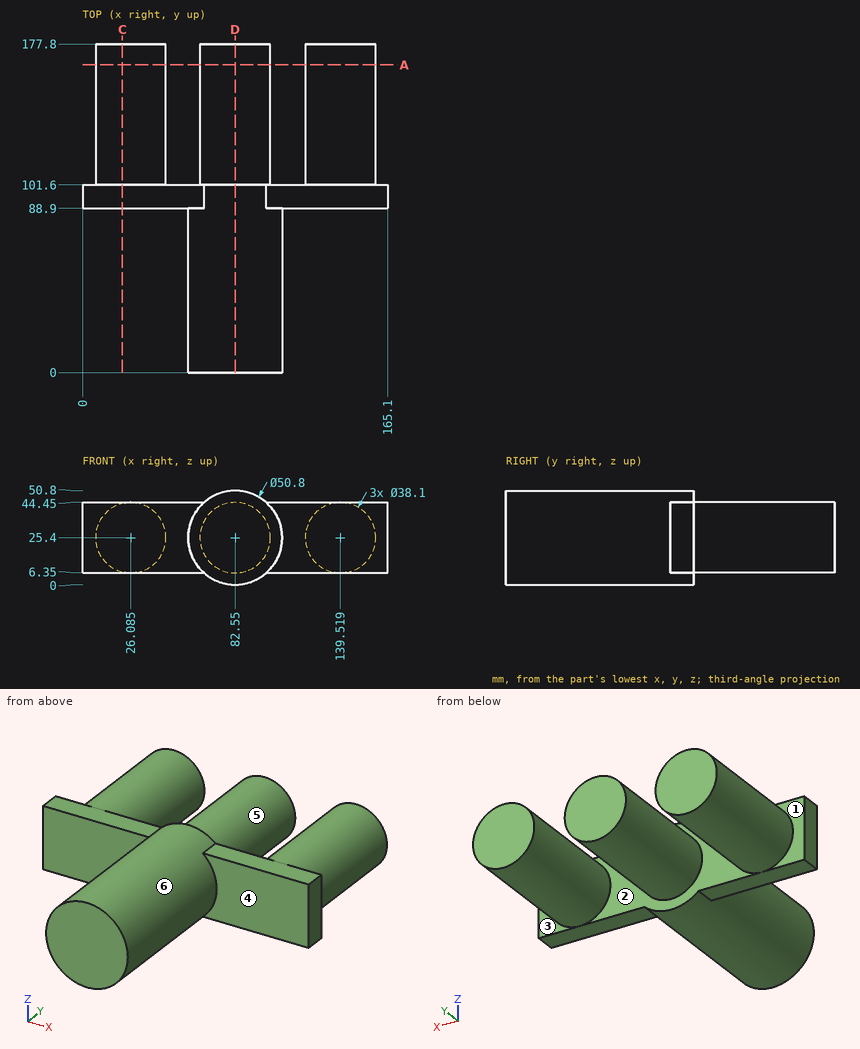
Geometry: see drawing. Coordinates: mm, zero at the bounding-box minimum. A direction names the side the tool comes from. Coordinates: 2 decimals unless noted, no trailing zeros. Write each loop counter-clockwise with the first axis right and the second up, starting at its lowest first coordinate (ties: lowest second). Pieces come first, ordered by that corner, then holes.
1) Section A-A on y = 166.5. State how many separate pieces and enclosed holes the cut face has, and give its area (3 significant figures).
2) Section D-D on x = 82.55. Output: boundary loops of the cut face in (y, z), and give its area (3 significant figures).
3) Section C-C on x = 21.5. Output: boundary loops of the cut face in (y, z).
4) Set-up query: the marked faces 1, 2 and 3. Return all of +Z, -Z, +X, -X, +Y, -Y with unobstructed straight access to the full face (end or side cutting, diameter ignored); none if empty.
5) Mould query, pull axis X, two halves, no side actions, for the marked faces 4, 5 and 6. Classes: pulls with the +X half, pulls with the -X half, needs draft (parallel to the pull), parting line crosses it, or undercut.
6) Material intervals for line 1 along X through (y, z) = (110, 39.5) (1 decimal); line 2 along X through (y, z) = (162, 17) (1 decimal); line 3 along Y through (x, z) = (157, 8), sorted ascending.
7) Pin query (flat end, axial travel): pin 1 Ø15 at (x, z) = (55.5, 27) entering from +Y; pin 2 Ø4 at (x, y) = (124.5, 97.5) entering from +Z; pin 3 Ø14 at (x, y) = (142, 92.5) entering from -Z. Return the tip coordinate at first contact, or that it passes through.
Check result:
1. separate pieces: 3
1. enclosed holes: 0
1. area: 3,420 mm2
2. outline: (0, 0) - (101.6, 0) - (101.6, 6.35) - (177.8, 6.35) - (177.8, 44.45) - (101.6, 44.45) - (101.6, 50.8) - (0, 50.8) - close
2. area: 8,060 mm2
3. outline: (88.9, 6.35) - (101.6, 6.35) - (101.6, 6.91) - (177.8, 6.91) - (177.8, 43.89) - (101.6, 43.89) - (101.6, 44.45) - (88.9, 44.45) - close
4. face 1: -X, +Y
4. face 2: +Y
4. face 3: +X, +Y
5. face 4: needs draft
5. face 5: undercut
5. face 6: parting line crosses it
6. line 1: x = 13.3 to 38.9, 69.7 to 95.4, 126.7 to 152.3
6. line 2: x = 9 to 43.2, 65.5 to 99.6, 122.4 to 156.6
6. line 3: y = 88.9 to 101.6
7. pin 1: stops at y = 101.6
7. pin 2: stops at z = 44.45
7. pin 3: stops at z = 6.35
